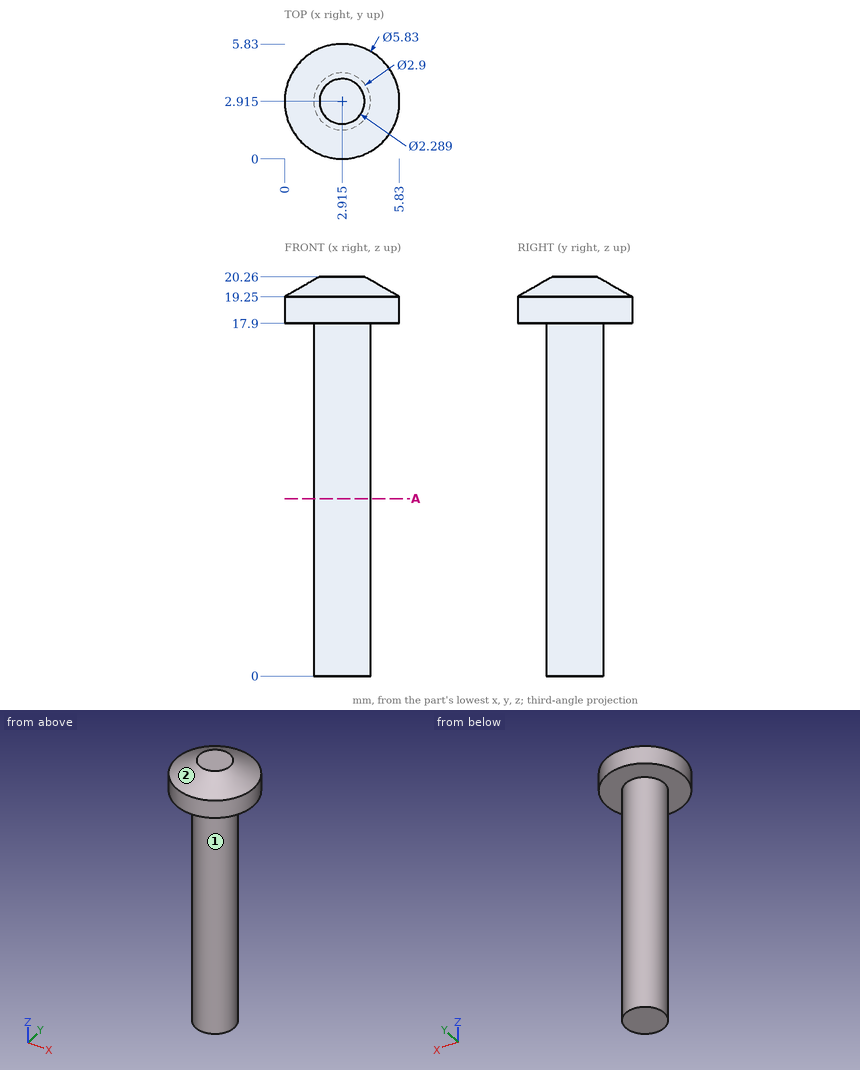
Check sheet for the drawn part. Datum: minimum x, y, z corner. Units: mm. A direction names the side the tool comes from. Round coordinates to 2 decimals unless told otherwise and drop trailing zeros. Loops run counter-clockwise (first coordinate to the right, second up) from the corner with the lowest first, then second, coordinate; pieces in that order, holes last.
Item 1: Gauge pin test, flat ends, axial feed: pin 1 (2 mm diameter, centred on y = 3.5, z = 7.5, fed in from -X) (3 decimals); pin 2 (1 mm diameter, centred on x = 4.5, y = 1.5, fed in from -Z); pin 3 (1.5 mm diameter, centred on x = 2, z = 11.5, fed in from -Y). Record the tip position at first contact, or that the pin passes through.
Item 2: Access from +Z, -Z, +X, -X, +Y, -Y to the whole of each face (thin tool, end or side, straight path). Record for the marked faces 1 and 2.
Item 3: Thickness scan on line 1 (X direction, y = 2.75, z = 18) (1 decimal); line 2 (Y direction, x = 3, z = 17.5); line 3 (X direction, y = 3.15, z = 13.25). Record the ranges inside material, lowest first.
Item 4: Cross-section at A-A on z = 9. Record the boundary of the cut face in (x, y) (3 decimals).
Answer sheet:
1. pin 1: stops at x = 1.465
1. pin 2: stops at z = 17.9
1. pin 3: stops at y = 1.47
2. face 1: -Z
2. face 2: +Z
3. line 1: x = 0 to 5.8
3. line 2: y = 1.47 to 4.36
3. line 3: x = 1.48 to 4.35
4. outline: circle Ø2.9 at (2.915, 2.915)
